Design review of the part built by this model. Coordinates are the model's own, in mm. Give positions to 0.01 mm unless a question says otherwise; leave off trailing zeros. Loops run counter-clockwise (first coordinate to the right, second up) from the corner with the lowest first, then second, coordinate; pieces in that order, holes last. Notation, with made-up numbers: (-16.5, -21) -> (29.5, -21) arc R20 cw to (29.5, 14) -> close; hole circle Ø9 at (-15, 72.25). An arc over 180 degrees is marked (long way). Answer as CSV lines item,"result".
from build123d import *

# Parameters (mm, degrees)
F1_DEPTH       = 3
F2_R           = 1
F4_D           = 3.3
F4_CSINK_D     = 6.72
F4_CSINK_ANGLE = 90
F5_W           = 40.2
F5_H           = 40.2
F6_DEPTH       = 0.5


with BuildPart() as f1:
    # F0 (on Top) → F1 (new body)
    with BuildSketch(Plane.XY):
        with BuildLine():
            Line((-28, -29), (28, -29))
            ThreePointArc((28, -29), (28.7071067812, -28.7071067812), (29, -28))
            Line((29, -28), (29, 28))
            ThreePointArc((29, 28), (28.7071067812, 28.7071067812), (28, 29))
            Line((28, 29), (-28, 29))
            ThreePointArc((-28, 29), (-28.7071067812, 28.7071067812), (-29, 28))
            Line((-29, 28), (-29, -28))
            ThreePointArc((-29, -28), (-28.7071067812, -28.7071067812), (-28, -29))
        make_face()
    extrude(amount=F1_DEPTH)

    # F2
    f2_edges = [f1.edges().sort_by_distance(p)[0] for p in [
        (29, 0, 3),
    ]]
    fillet(f2_edges, radius=F2_R)

    # F4 (through all)
    with Locations(Plane.XY.offset(3)):
        with Locations((-24, 24), (24, 24), (-24, -24), (24, -24)):
            CounterSinkHole(F4_D / 2, F4_CSINK_D / 2, counter_sink_angle=F4_CSINK_ANGLE)

    # F5 (on face) → F6 (cut)
    with BuildSketch(Plane.XY.offset(3)):
        Rectangle(F5_W, F5_H)
    extrude(amount=-F6_DEPTH, mode=Mode.SUBTRACT)


solid = f1.part
Q1. We need section C-C, the plane y = -10. State the section outline as (x, z) points, and give its area (3 significant figures).
Filled sheet:
outline,"(-29, 0) -> (29, 0) -> (29, 2) arc R1 ccw to (28, 3) -> (20.1, 3) -> (20.1, 2.5) -> (-20.1, 2.5) -> (-20.1, 3) -> (-28, 3) arc R1 ccw to (-29, 2) -> close"
area,"153 mm^2"
Q2. Clearance check with flat-ended pins moving along their axes: pin 1 Ø4.5 at (x, y) = (-24, 24) entering from +Z; pin 2 Ø12 at (x, y) = (-3.5, -6.5) entering from +Z; pin 3 Ø2 at (x, y) = (24, 24) entering from +Z; pin 4 Ø0.6 at (x, z) = (9, 3) entering from -Y. State where each tip first meets the part, or that it passes through.
Filled sheet:
pin 1,"stops at z = 1.89"
pin 2,"stops at z = 2.5"
pin 3,"passes through"
pin 4,"stops at y = -28.71"
Q3. The part is to be moulded in two halves that separate along X. For faces 1 (the cylindrical face through (25.216, 25.115, 0.636)), 2 (the flat face through (0, -21, 3)), 3 (the flat face through (0, 0, 2.5)), 4 (the flat face through (29, 0, 1)), say which applies: pulls with the +X half, pulls with the -X half, needs draft (parallel to the pull), parting line crosses it, or undercut.
Filled sheet:
face 1,"undercut"
face 2,"needs draft"
face 3,"undercut"
face 4,"pulls with the +X half"
Q4. We need section A-A, the plane x = -24. State the section outline as (y, z) points, and give its area (3 significant figures).
Filled sheet:
outline,"(-29, 0) -> (-25.65, 0) -> (-25.65, 1.29) -> (-27.36, 3) -> (-28, 3) arc R1 ccw to (-29, 2) -> close; (-22.35, 0) -> (22.35, 0) -> (22.35, 1.29) -> (20.64, 3) -> (-20.64, 3) -> (-22.35, 1.29) -> close; (25.65, 0) -> (29, 0) -> (29, 2) arc R1 ccw to (28, 3) -> (27.36, 3) -> (25.65, 1.29) -> close"
area,"148 mm^2"
Q5. To check wall thickness, follow probe 1 along X at (y, z) = (24, 0.6); probe 2 along X at (y, z) = (-24.5, 2). State the ranges of each line that lie inside material, in increasing order. Write a range as from..to.
Filled sheet:
probe 1,"x = -29..-25.65, -22.35..22.35, 25.65..29"
probe 2,"x = -29..-26.31, -21.69..21.69, 26.31..29"
